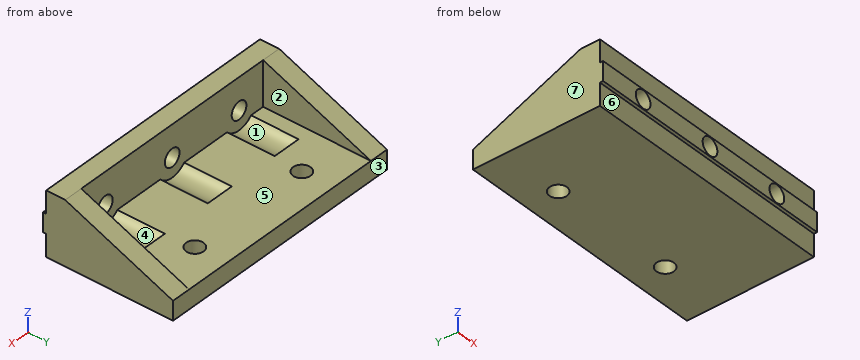
from build123d import *

# Parameters (mm, degrees)
CROQUIS1_W                 = 80
CROQUIS1_H                 = 40
SALIENTE_EXTRUIR1_DEPTH    = 20
CROQUIS2_W                 = 68
CROQUIS2_H                 = 14
CORTAR_EXTRUIR1_DEPTH      = 34
CORTAR_EXTRUIR2_DEPTH      = 80
CORTAR_EXTRUIR3_REACH      = 22
CROQUIS4_R                 = 2.75
CROQUIS8_W                 = 80
CROQUIS8_H                 = 6
SALIENTE_EXTRUIR2_DEPTH    = 1
CROQUIS5_R                 = 2.75
CORTAR_EXTRUIR6_DEPTH      = 2
CORTAR_EXTRUIR6_DEPTH_BACK = 41
CROQUIS9_R                 = 6
CORTAR_EXTRUIR8_DEPTH      = 15


with BuildPart() as part:
    # Croquis1 → Saliente-Extruir1 (new body)
    with BuildSketch(Plane.XY):
        with Locations((40, -20)):
            Rectangle(CROQUIS1_W, CROQUIS1_H)
    extrude(amount=SALIENTE_EXTRUIR1_DEPTH)

    # Croquis2 → Cortar-Extruir1 (cut)
    with BuildSketch(Plane(origin=(0, 0, 0), x_dir=(1, 0, 0), z_dir=(0, 1, 0))):
        with Locations((40, -13)):
            Rectangle(CROQUIS2_W, CROQUIS2_H)
    extrude(amount=-CORTAR_EXTRUIR1_DEPTH, mode=Mode.SUBTRACT)

    # Croquis3 → Cortar-Extruir2 (cut)
    with BuildSketch(Plane.ZY):
        Polygon((20, 0), (20, -34), (6, 0), align=None)
    extrude(amount=-CORTAR_EXTRUIR2_DEPTH, mode=Mode.SUBTRACT)

    # Croquis4 → Cortar-Extruir3 (cut, up to next)
    with BuildSketch(Plane(origin=(0, 0, 0), x_dir=(-1, 0, 0), z_dir=(0, 0, -1)), mode=Mode.PRIVATE) as cortar_extruir3_sk1:
        with Locations((-60, -10)):
            Circle(CROQUIS4_R)
    cortar_extruir3_tool1 = extrude(cortar_extruir3_sk1.sketch, amount=-CORTAR_EXTRUIR3_REACH, mode=Mode.PRIVATE) & part.part
    add(cortar_extruir3_tool1.solids().sort_by_distance((60, -10, 0))[0], mode=Mode.SUBTRACT)
    # Croquis4 → Cortar-Extruir3 (cut, up to next)
    with BuildSketch(Plane(origin=(0, 0, 0), x_dir=(-1, 0, 0), z_dir=(0, 0, -1)), mode=Mode.PRIVATE) as cortar_extruir3_sk2:
        with Locations((-20, -10)):
            Circle(CROQUIS4_R)
    cortar_extruir3_tool2 = extrude(cortar_extruir3_sk2.sketch, amount=-CORTAR_EXTRUIR3_REACH, mode=Mode.PRIVATE) & part.part
    add(cortar_extruir3_tool2.solids().sort_by_distance((20, -10, 0))[0], mode=Mode.SUBTRACT)

    # Croquis8 → Saliente-Extruir2 (add)
    with BuildSketch(Plane.XZ.offset(40)):
        with Locations((40, 10)):
            Rectangle(CROQUIS8_W, CROQUIS8_H)
    extrude(amount=SALIENTE_EXTRUIR2_DEPTH)

    # Croquis5 → Cortar-Extruir6 (cut, two sides)
    with BuildSketch(Plane.XZ.offset(40)) as cortar_extruir6_sk:
        with Locations((15, 10)):
            Circle(CROQUIS5_R)
        with Locations((40, 10)):
            Circle(CROQUIS5_R)
        with Locations((65, 10)):
            Circle(CROQUIS5_R)
    extrude(amount=CORTAR_EXTRUIR6_DEPTH, mode=Mode.SUBTRACT)
    extrude(cortar_extruir6_sk.sketch, amount=-CORTAR_EXTRUIR6_DEPTH_BACK, mode=Mode.SUBTRACT)

    # Croquis9 → Cortar-Extruir8 (cut)
    with BuildSketch(Plane(origin=(0, -34, 0), x_dir=(1, 0, 0), z_dir=(0, 1, 0))):
        with Locations((15, -10)):
            Circle(CROQUIS9_R)
        with Locations((40, -10)):
            Circle(CROQUIS9_R)
        with Locations((65, -10)):
            Circle(CROQUIS9_R)
    extrude(amount=CORTAR_EXTRUIR8_DEPTH, mode=Mode.SUBTRACT)


solid = part.part
Geometry check sheet. Reference: the model listing, model coordinates, mm. Face numbers are marked on the shaded views. A direction names the side the tool comes from. Give positions to 0.01 mm unless a question says otherwise; leave off trailing zeros. Write each loop counter-clockwise with the first axis right and the second up, starting at its lowest first coordinate (ties: lowest second). Pieces come first, ordered by that corner, then holes. Notation, with made-up numbers: M -38.75,-11.5 L 20.25,-11.5 A16 ccw 20.25,10.5 Z; hole C -25.5,25 d10. An arc over 180 degrees is marked long. One line per question, with ' | ' between items.
1. Set-up check for the marked faces 4, 5, 6 and 7: record each of +Z, -Z, +X, -X, +Y, -Y from which the full face is reachable in a straight line by a thin tool's end or side.
Ans:
face 4: +Z | face 5: +Z, +Y | face 6: -Z, +X, -X, -Y | face 7: +Z, -Z, -X, +Y, -Y
2. Cross-section at A-A (x = 15). Enter the section's corners in (y, z).
Ans:
outline: M -41,7 L -40,7 L -40,0 L 0,0 L 0,6 L -19,6 L -19,4 L -34,4 L -34,7.25 L -41,7.25 Z; M -41,12.75 L -34,12.75 L -34,20 L -40,20 L -40,13 L -41,13 Z
3. Gauge pin test, flat ends, axial feed: pin 1 (1 mm diameter, centred on x = 32, y = -6, fed in from +Z); pin 2 (1.5 mm diameter, centred on x = 36.5, y = -14, fed in from -Z); pin 3 (6.5 mm diameter, centred on x = 15, z = 10, fed in from +Y); pin 4 (0.5 mm diameter, centred on x = 41.5, y = -40.5, fed in from -Z). Record the tip position at first contact, or that the pin passes through.
Ans:
pin 1: z = 6 | pin 2: z = 0 | pin 3: y = -34 | pin 4: z = 7
4. Scan lines: line 1 along X through (y, z) = (-36.75, 10); line 2 along X through (y, z) = (-27, 6.5); line 3 along Z through (x, y) = (65, -36.75). Record each from-to range of solid material in increasing order. Write a range as from..to.
Ans:
line 1: 0..12.25, 17.75..37.25, 42.75..62.25, 67.75..80 | line 2: 0..6, 74..80 | line 3: 0..7.25, 12.75..20
5. Cross-section at B-B (y = -10). Enter the section's corners in (x, z), plus the area to 3 significant figures.
Ans:
outline: M 0,0 L 17.25,0 L 17.25,6 L 6,6 L 6,10.12 L 0,10.12 Z; M 22.75,0 L 57.25,0 L 57.25,6 L 22.75,6 Z; M 62.75,0 L 80,0 L 80,10.12 L 74,10.12 L 74,6 L 62.75,6 Z | area: 463 mm2
6. Mould release check, pull along Y, two halves, no side actions. Record for the marked faces 1, 2 and 3: released by +Y, released by -Y, zero draft, split by the parting line, or undercut.
Ans:
face 1: undercut | face 2: zero draft | face 3: released by +Y
7. Cross-section at D-D (y = -26.5). Enter the section's corners in (x, z), plus the area to 3 significant figures.
Ans:
outline: M 0,0 L 80,0 L 80,16.91 L 74,16.91 L 74,6 L 69.47,6 A6 cw 60.53,6 L 44.47,6 A6 cw 35.53,6 L 19.47,6 A6 cw 10.53,6 L 6,6 L 6,16.91 L 0,16.91 Z | area: 574 mm2
8. Cross-section at C-C (z = 10). Enter the section's corners in (x, y), plus the area to 3 significant figures.
Ans:
outline: M 0,-41 L 12.25,-41 L 12.25,-34 L 6,-34 L 6,-9.71 L 0,-9.71 Z; M 17.75,-41 L 37.25,-41 L 37.25,-34 L 17.75,-34 Z; M 42.75,-41 L 62.25,-41 L 62.25,-34 L 42.75,-34 Z; M 67.75,-41 L 80,-41 L 80,-9.71 L 74,-9.71 L 74,-34 L 67.75,-34 Z | area: 736 mm2
